Geometry check sheet. Reference: drawing and pictorial views, mm from the part's lowest x, y, z. A direction names the side the tool comes from. Coordinates: 2 decimals unless noted, no trailing zeros. Write each loop counter-clockwise with the first axis right and the second up, starting at its lowest first coordinate (ties: lowest second). Pieces come first, ordered by that corner, then holes. Notation, with made-up numbers: (66.5, 82.5) - (124.5, 82.5) arc R17 ccw to (124.5, 104.5) - close; hole circle Ø3 at (86, 13). An arc over 180 degrees is marked (long way). Use one line per item in the form item = value. Start each with the question number.
(1) Sectioned sample at B-B (z = 54.5). Record the cut outline in (x, y).
(2) Mould release check, pull along Y, two halves, no side actions. Record for the marked faces 1, 2 and 3: released by +Y, released by -Y, zero draft, split by the parting line, or undercut.
(3) Sectioned sample at D-D (x = 85). Record the cut outline in (y, z).
(4) Sectioned sample at C-C (x = 13.5). Record the cut outline in (y, z), and give its area (3 significant figures).
(5) Tool access check on the marked faces 4, 5, 6, 7 and 8. Record the directions out of +Z, -Z, +X, -X, +Y, -Y that give a thin tool (end or side, any length) a straight path to the whole face; none if there is none.
(6) Gauge pin test, flat ends, axial feed: pin 1 Ø5 at (x, z) = (46, 44) entering from -Y; pin 2 Ø21.5 at (y, z) = (33.5, 26) entering from +X. Record the tip position at first contact, or that the pin passes through.
(7) Material ranges on line 1 (Z direction, x = 11.5, y = 29); line 2 (Y direction, x = 13, z = 13); line 3 (X direction, y = 73.5, z = 16), recorded low to high. Write a range as [from, to].
(8) Sectioned sample at A-A (y = 40.5). Record the cut outline in (x, z), and give its area (3 significant figures).
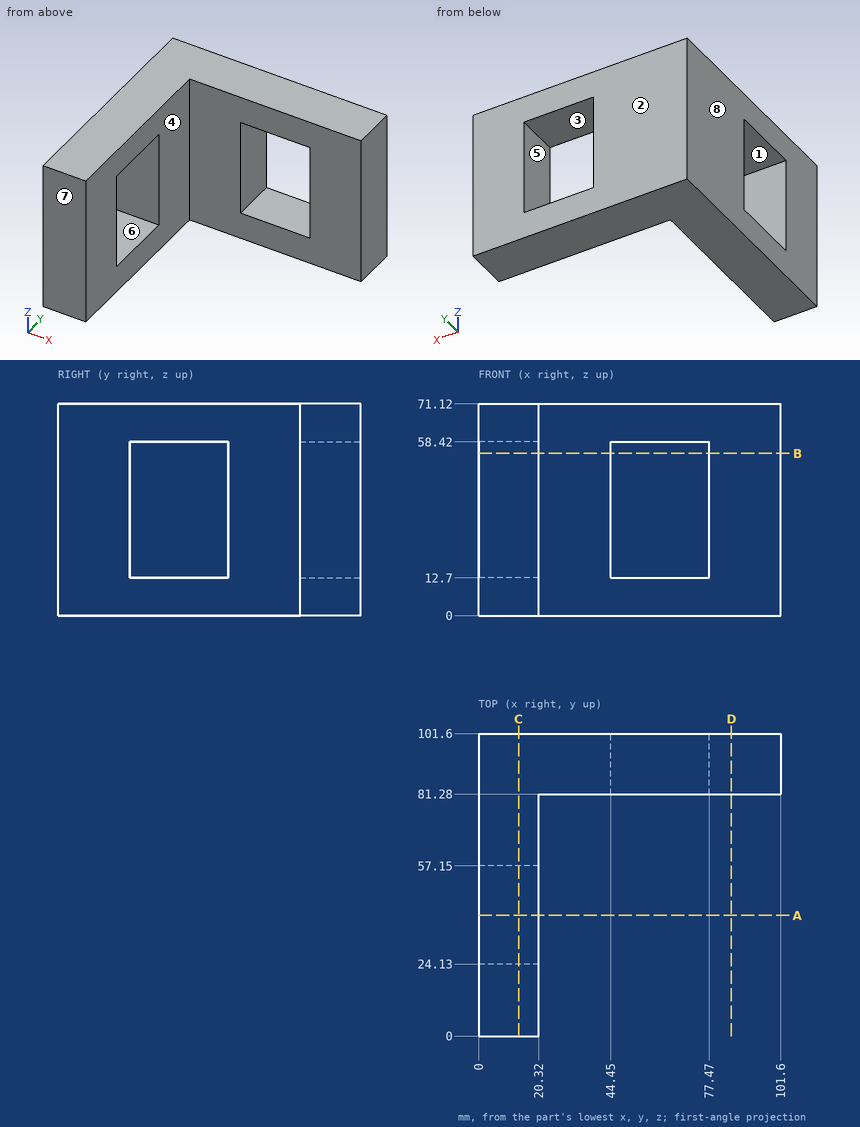
Answers below:
q1.outline = (0, 0) - (20.32, 0) - (20.32, 24.13) - (0, 24.13) - close; (0, 57.15) - (20.32, 57.15) - (20.32, 81.28) - (44.45, 81.28) - (44.45, 101.6) - (0, 101.6) - close; (77.47, 81.28) - (101.6, 81.28) - (101.6, 101.6) - (77.47, 101.6) - close
q2.face_1 = undercut
q2.face_2 = released by +Y
q2.face_3 = zero draft
q3.outline = (81.28, 0) - (101.6, 0) - (101.6, 71.12) - (81.28, 71.12) - close
q4.outline = (0, 0) - (101.6, 0) - (101.6, 71.12) - (0, 71.12) - close; hole (24.13, 12.7) - (57.15, 12.7) - (57.15, 58.42) - (24.13, 58.42) - close
q4.area = 5,720 mm2
q5.face_4 = +Z, -Z, +X, -Y
q5.face_5 = +Y, -Y
q5.face_6 = +X, -X
q5.face_7 = +Z, -Z, +X, -X, -Y
q5.face_8 = +Z, -Z, -X, +Y, -Y
q6.pin_1 = 81.28
q6.pin_2 = 20.32
q7.line_1 = [0, 12.7], [58.42, 71.12]
q7.line_2 = [0, 24.13], [57.15, 101.6]
q7.line_3 = [0, 20.32]
q8.outline = (0, 0) - (20.32, 0) - (20.32, 12.7) - (0, 12.7) - close; (0, 58.42) - (20.32, 58.42) - (20.32, 71.12) - (0, 71.12) - close
q8.area = 516 mm2
